```python
from build123d import *

# Parameters (mm, degrees)
F0_W     = 117
F0_H     = 92.5
F1_DEPTH = 2.5
F2_W     = 2.5
F2_H     = 90
F3_DEPTH = 50
F2_W_2   = 47
F2_H_2   = 28
F4_DEPTH = 25
F5_R     = 1.75
F6_DEPTH = 25
F7_R     = 2.49999
F8_W     = 57.49999
F8_H     = 2.5
F8_W_2   = 87.50001
F9_DEPTH = 15
F10_R    = 5


# Not quite as in the source:
# - a fillet or chamfer is up to 0.001 mm smaller than in the source, because OpenCascade refuses the exact size


with BuildPart() as f1:
    # F0 (on Top) → F1 (new body)
    with BuildSketch(Plane.XY):
        with Locations((0, 6.6284866768)):
            Rectangle(F0_W, F0_H)
    extrude(amount=F1_DEPTH)

    # F2 (on face) → F3 (join)
    with BuildSketch(Plane.XY.offset(2.5)):
        with Locations((57.25, 7.8784866768)):
            Rectangle(F2_W, F2_H)
        Polygon((-58.5, -37.1215133232), (-58.5, -39.6215133232), (58.5, -39.6215133232), (58.5, -37.1215133232), (56, -37.1215133232), (-56, -37.1215133232), align=None)
        with Locations((-57.25, 7.8784866768)):
            Rectangle(F2_W, F2_H)
    extrude(amount=F3_DEPTH)

    # F2 (on face) → F4 (cut)
    with BuildSketch(Plane.XY.offset(2.5)):
        with Locations((-22.5, -15.6215133232)):
            Rectangle(F2_W_2, F2_H_2)
    extrude(amount=-F4_DEPTH, mode=Mode.SUBTRACT)

    # F5 (on face) → F6 (cut)
    with BuildSketch(Plane(origin=(-58.5, 0, 0), x_dir=(0, -1, 0), z_dir=(-1, 0, 0))):
        with Locations((-42.8784866768, 27.5)):
            Circle(F5_R)
    extrude(amount=-F6_DEPTH, mode=Mode.SUBTRACT)

    # F7 (radius 2.5 in the source; OpenCascade refuses exactly that, so slightly less here)
    f7_edges = [f1.edges().sort_by_distance(p)[0] for p in [
        (-58.5, 6.628487, 0),
        (-58.5, -39.621513, 26.25),
        (0, -39.621513, 0),
        (58.5, 6.628487, 0),
        (58.5, -39.621513, 26.25),
        (0, 52.878487, 0),
        (-58.5, 52.878487, 26.25),
        (58.5, 52.878487, 26.25),
    ]]
    fillet(f7_edges, radius=F7_R)

    # F8 (on face) → F9 (join)
    with BuildSketch(Plane.YZ.offset(58.5)):
        with Locations((79.1284916768, 51.25)):
            Rectangle(F8_W, F8_H)
        with Locations((6.6284916768, 51.25)):
            Rectangle(F8_W_2, F8_H)
    extrude(amount=F9_DEPTH)

    # F10
    f10_edges = [f1.edges().sort_by_distance(p)[0] for p in [
        (73.5, 107.878487, 51.25),
        (58.5, 107.878487, 51.25),
        (73.5, -37.121513, 51.25),
    ]]
    fillet(f10_edges, radius=F10_R)


solid = f1.part
```
Input: part model. Units: mm. Frame: model coordinates. A direction names the side the tool comes from. Coordinates: 2 decimals unless noted, no trailing zeros. One line per item, written item: value.
(1) Line query: line 1 along X through (y, z) = (35, 18); line 2 along Y through (x, z) = (-19, 29.5); line 3 along Z through (x, y) = (8.5, 13.5). Output: solid intervals per line, ascending. Write a range as from..to.
Filled in:
line 1: -58.5..-56, 56..58.5
line 2: -39.62..-37.12
line 3: 0..2.5
(2) Pin query (flat end, axial travel): pin 1 (2 mm diameter, centred on y = 42.88, z = 27.5, fed in from -X); pin 2 (25 mm diameter, centred on y = -6.5, z = 22.5, fed in from +X); pin 3 (16.5 mm diameter, centred on x = 67, y = 9.5, fed in from -Z). Return the tip coordinate at first contact, or that it passes through.
Filled in:
pin 1: x = 56
pin 2: x = 58.5
pin 3: z = 50
(3) Reachability of faces 4 (the flat face through (-1, 9, 2.5)), 5 (the flat face through (-58.5, 7, 27)), 6 (the flat face through (58.5, 6, 27)) from +Z, -Z, +X, -X, +Y, -Y: full face, straight path, thin tool, end or side. Return the list, or none.
Filled in:
face 4: +Z, +Y
face 5: +Z, -Z, -X, +Y, -Y
face 6: -Z, +X, +Y, -Y
(4) Pull-direction query (Y, two-part tool) for faces 1 (the cylindrical face through (60, 106.45, 51.27)), 2 (the cylindrical face through (-57.3, 41.2, 28)), 3 (the flat face through (66, 34, 50)); classes: +Y half, -Y half, draft (parallel to the pull), parting line (faces both ways), or undercut.
Filled in:
face 1: +Y half
face 2: undercut
face 3: draft
